Can you work these out from the model? Positions are in its coordinate system, mm. A direction names the side the tool comes from. Give positions to 0.01 mm unless a question says otherwise; leave off trailing zeros. Loops run counter-clockwise (first coordinate to the right, second up) from the corner with the lowest first, then second, coordinate; pieces in that order, holes last. Notation, with made-up numbers: (25, -3.75) - (79, -3.75) arc R27 cw to (79, 26.25) - close; hole circle Ø8 at (34.5, 0). An arc over 180 degrees is marked (long way). Answer as a JSON object with one key per item and string values.
```python
from build123d import *

# Parameters (mm, degrees)
EXTRUDE_1_DEPTH      = 8
SKETCH_2_R           = 2
CUT_EXTRUDE_1_DEPTH  = 8
SKETCH_3_W           = 235.5
SKETCH_3_H           = 139.5
CUT_EXTRUDE_2_DEPTH  = 6
SKETCH_4_R           = 2
CUT_EXTRUDE_3_DEPTH  = 6
SKETCH_6_W           = 6
SKETCH_6_H           = 6
SKETCH_6_R           = 2.1
EXTRUDE_2_DEPTH      = 4
SKETCH_7_R           = 24
SKETCH_7_R_2         = 21.5
EXTRUDE_3_DEPTH      = 3
SKETCH_8_R           = 2
CUT_EXTRUDE_4_DEPTH  = 3
SKETCH_9_W           = 11.5
SKETCH_9_H           = 15.5
CUT_EXTRUDE_5_DEPTH  = 7
CUT_EXTRUDE_6_DEPTH  = 6
SKETCH_11_W          = 20
SKETCH_11_H          = 26.5
CUT_EXTRUDE_8_DEPTH  = 1
SKETCH_13_W          = 26.5
SKETCH_13_H          = 5.5
CUT_EXTRUDE_9_DEPTH  = 5.25
SKETCH_14_W          = 9.2
SKETCH_14_H          = 3.5
SKETCH_14_W_2        = 7.8
SKETCH_14_H_2        = 1
CUT_EXTRUDE_10_DEPTH = 5.25
EXTRUDE_5_DEPTH      = 5.25
EXTRUDE_6_DEPTH      = 5.25
SKETCH_17_R          = 3
CUT_EXTRUDE_11_DEPTH = 2


with BuildPart() as part:
    # 草图1 → 凸台-拉伸1 (new body)
    with BuildSketch(Plane(origin=(0, 0, 0), x_dir=(1, 0, 0), z_dir=(0, 1, 0))):
        with BuildLine():
            Line((-106.707018927, 68.788249211), (123.292981073, 68.788249211))
            ThreePointArc((123.292981073, 68.788249211), (130.364048884, 65.859317023), (133.292981073, 58.788249211))
            Line((133.292981073, 58.788249211), (133.292981073, -80.961750789))
            ThreePointArc((133.292981073, -80.961750789), (130.364048884, -88.032818601), (123.292981073, -90.961750789))
            Line((123.292981073, -90.961750789), (-106.707018927, -90.961750789))
            ThreePointArc((-106.707018927, -90.961750789), (-113.778086739, -88.032818601), (-116.707018927, -80.961750789))
            Line((-116.707018927, -80.961750789), (-116.707018927, 58.788249211))
            ThreePointArc((-116.707018927, 58.788249211), (-113.778086739, 65.859317023), (-106.707018927, 68.788249211))
        make_face()
    extrude(amount=EXTRUDE_1_DEPTH)

    # 草图2 → 切除-拉伸1 (cut)
    with BuildSketch(Plane(origin=(0, 8, 0), x_dir=(1, 0, 0), z_dir=(0, 1, 0))):
        with Locations(Location((-103.707018927, 63.788249211, 0), (0, 0, 270))):
            Circle(SKETCH_2_R)
        with Locations(Location((-103.707018927, -85.961750789, 0), (0, 0, 270))):
            Circle(SKETCH_2_R)
        with Locations(Location((120.292981073, -85.961750789, 0), (0, 0, 270))):
            Circle(SKETCH_2_R)
        with Locations(Location((120.292981073, 63.788249211, 0), (0, 0, 270))):
            Circle(SKETCH_2_R)
    extrude(amount=-CUT_EXTRUDE_1_DEPTH, mode=Mode.SUBTRACT)

    # 草图3 → 切除-拉伸2 (cut)
    with BuildSketch(Plane(origin=(0, 8, 0), x_dir=(1, 0, 0), z_dir=(0, 1, 0))):
        with Locations((9.292981073, -11.211750789)):
            Rectangle(SKETCH_3_W, SKETCH_3_H)
    extrude(amount=-CUT_EXTRUDE_2_DEPTH, mode=Mode.SUBTRACT)

    # 草图4 → 切除-拉伸3 (cut)
    with BuildSketch(Plane(origin=(0, 2, 0), x_dir=(1, 0, 0), z_dir=(0, 1, 0))):
        with Locations(Location((-25.957018927, 40.538249211, 0), (0, 0, 270))):
            Circle(SKETCH_4_R)
        with Locations(Location((-7.957018927, 40.538249211, 0), (0, 0, 270))):
            Circle(SKETCH_4_R)
        with Locations(Location((10.042981073, 40.538249211, 0), (0, 0, 270))):
            Circle(SKETCH_4_R)
        with Locations(Location((28.042981073, 40.538249211, 0), (0, 0, 270))):
            Circle(SKETCH_4_R)
        with Locations(Location((50.042981073, 40.538249211, 0), (0, 0, 270))):
            Circle(SKETCH_4_R)
    extrude(amount=-CUT_EXTRUDE_3_DEPTH, mode=Mode.SUBTRACT)

    # 草图6 → 凸台-拉伸2 (add)
    # profile 1 of 3: a face of its own
    with BuildSketch(Plane(origin=(0, 2, 0), x_dir=(1, 0, 0), z_dir=(0, 1, 0))):
        with Locations((58.042981073, 40.538249211)):
            Rectangle(SKETCH_6_W, SKETCH_6_H)
        with Locations(Location((58.042981073, 40.538249211, 0), (0, 0, 270))):
            Circle(SKETCH_6_R, mode=Mode.SUBTRACT)
    # profile 2 of 3: a face of its own
    with BuildSketch(Plane(origin=(0, 2, 0), x_dir=(1, 0, 0), z_dir=(0, 1, 0))):
        with Locations((1.042981073, 40.538249211)):
            Rectangle(SKETCH_6_W, SKETCH_6_H)
        with Locations(Location((1.042981073, 40.538249211, 0), (0, 0, 270))):
            Circle(SKETCH_6_R, mode=Mode.SUBTRACT)
    # profile 3 of 3: a face of its own
    with BuildSketch(Plane(origin=(0, 2, 0), x_dir=(1, 0, 0), z_dir=(0, 1, 0))):
        with Locations((-34.957018927, 40.538249211)):
            Rectangle(SKETCH_6_W, SKETCH_6_H)
        with Locations(Location((-34.957018927, 40.538249211, 0), (0, 0, 270))):
            Circle(SKETCH_6_R, mode=Mode.SUBTRACT)
    extrude(amount=EXTRUDE_2_DEPTH)

    # 草图7 → 凸台-拉伸3 (add)
    # profile 1 of 2: a face of its own
    with BuildSketch(Plane(origin=(0, 2, 0), x_dir=(1, 0, 0), z_dir=(0, 1, 0))):
        with Locations(Location((-76.707018927, 28.788249211, 0), (0, 0, 270))):
            Circle(SKETCH_7_R)
        with Locations(Location((-76.707018927, 28.788249211, 0), (0, 0, 270))):
            Circle(SKETCH_7_R_2, mode=Mode.SUBTRACT)
    # profile 2 of 2: a face of its own
    with BuildSketch(Plane(origin=(0, 2, 0), x_dir=(1, 0, 0), z_dir=(0, 1, 0))):
        with Locations(Location((93.292981073, 28.788249211, 0), (0, 0, 270))):
            Circle(SKETCH_7_R)
        with Locations(Location((93.292981073, 28.788249211, 0), (0, 0, 270))):
            Circle(SKETCH_7_R_2, mode=Mode.SUBTRACT)
    extrude(amount=EXTRUDE_3_DEPTH)

    # 草图8 → 切除-拉伸4 (cut)
    with BuildSketch(Plane(origin=(0, 2, 0), x_dir=(1, 0, 0), z_dir=(0, 1, 0))):
        with Locations(Location((-82.480521619, 38.788249211, 0), (0, 0, 270))):
            Circle(SKETCH_8_R)
        with Locations(Location((-70.933516236, 38.788249211, 0), (0, 0, 270))):
            Circle(SKETCH_8_R)
        with Locations(Location((-65.160013544, 28.788249211, 0), (0, 0, 270))):
            Circle(SKETCH_8_R)
        with Locations(Location((-70.933516236, 18.788249211, 0), (0, 0, 270))):
            Circle(SKETCH_8_R)
        with Locations(Location((-82.480521619, 18.788249211, 0), (0, 0, 270))):
            Circle(SKETCH_8_R)
        with Locations(Location((-88.254024311, 28.788249211, 0), (0, 0, 270))):
            Circle(SKETCH_8_R)
        with Locations(Location((87.519478381, 38.788249211, 0), (0, 0, 270))):
            Circle(SKETCH_8_R)
        with Locations(Location((99.066483764, 38.788249211, 0), (0, 0, 270))):
            Circle(SKETCH_8_R)
        with Locations(Location((104.839986456, 28.788249211, 0), (0, 0, 270))):
            Circle(SKETCH_8_R)
        with Locations(Location((99.066483764, 18.788249211, 0), (0, 0, 270))):
            Circle(SKETCH_8_R)
        with Locations(Location((87.519478381, 18.788249211, 0), (0, 0, 270))):
            Circle(SKETCH_8_R)
        with Locations(Location((81.745975689, 28.788249211, 0), (0, 0, 270))):
            Circle(SKETCH_8_R)
    extrude(amount=-CUT_EXTRUDE_4_DEPTH, mode=Mode.SUBTRACT)

    # 草图9 → 切除-拉伸5 (cut)
    with BuildSketch(Plane(origin=(0, 8, 0), x_dir=(1, 0, 0), z_dir=(0, 1, 0))):
        with Locations((127.542981073, -43.211750789)):
            Rectangle(SKETCH_9_W, SKETCH_9_H)
    extrude(amount=-CUT_EXTRUDE_5_DEPTH, mode=Mode.SUBTRACT)

    # 草图10 → 切除-拉伸6 (cut)
    with BuildSketch(Plane(origin=(0, 8, 0), x_dir=(1, 0, 0), z_dir=(0, 1, 0))):
        Polygon((127.042981073, 33.788249211), (127.042981073, 22.788249211), (129.792981073, 22.788249211), (129.792981073, 17.788249211), (130.792981073, 17.788249211), (130.792981073, 24.788249211), (133.292981073, 24.788249211), (133.292981073, 31.788249211), (130.792981073, 31.788249211), (130.792981073, 38.788249211), (129.792981073, 38.788249211), (129.792981073, 33.788249211), align=None)
    extrude(amount=-CUT_EXTRUDE_6_DEPTH, mode=Mode.SUBTRACT)

    # 草图11 → 切除-拉伸8 (cut)
    with BuildSketch(Plane(origin=(0, 2, 0), x_dir=(1, 0, 0), z_dir=(0, 1, 0))):
        with Locations((122.292981073, -10.461750789)):
            Rectangle(SKETCH_11_W, SKETCH_11_H)
    extrude(amount=-CUT_EXTRUDE_8_DEPTH, mode=Mode.SUBTRACT)

    # 草图13 → 切除-拉伸9 (cut)
    with BuildSketch(Plane.ZY.offset(-127.042981073)):
        with Locations((10.461750789, 4.75)):
            Rectangle(SKETCH_13_W, SKETCH_13_H)
    extrude(amount=-CUT_EXTRUDE_9_DEPTH, mode=Mode.SUBTRACT)

    # 草图14 → 切除-拉伸10 (cut)
    with BuildSketch(Plane.ZY.offset(-132.292981073)):
        with Locations((15.611750789, 4.25)):
            Rectangle(SKETCH_14_W, SKETCH_14_H)
        with Locations((4.111750789, 3)):
            Rectangle(SKETCH_14_W_2, SKETCH_14_H_2)
    extrude(amount=-CUT_EXTRUDE_10_DEPTH, mode=Mode.SUBTRACT)

    # 草图15 → 凸台-拉伸5 (add)
    with BuildSketch(Plane.ZY.offset(-127.042981073)):
        Polygon((-2.788249211, 7.5), (-0.288249211, 7.5), (-2.788249211, 5), align=None)
    extrude(amount=-EXTRUDE_5_DEPTH)

    # 草图16 → 凸台-拉伸6 (add)
    with BuildSketch(Plane.ZY.offset(-127.042981073)):
        Polygon((23.711750789, 7.5), (23.711750789, 5.5), (21.711750789, 7.5), align=None)
    extrude(amount=-EXTRUDE_6_DEPTH)

    # 草图17 → 切除-拉伸11 (cut)
    with BuildSketch(Plane.XZ):
        with Locations(Location((-103.707018927, 85.961750789, 0), (0, 0, 270))):
            Circle(SKETCH_17_R)
        with Locations(Location((120.292981073, 85.961750789, 0), (0, 0, 270))):
            Circle(SKETCH_17_R)
        with Locations(Location((120.292981073, -63.788249211, 0), (0, 0, 270))):
            Circle(SKETCH_17_R)
        with Locations(Location((-103.707018927, -63.788249211, 0), (0, 0, 270))):
            Circle(SKETCH_17_R)
    extrude(amount=-CUT_EXTRUDE_11_DEPTH, mode=Mode.SUBTRACT)


solid = part.part
```
1) Imagine slicing it at B-B on x = -14.5. Write out the boundary of the cut face in (y, z), and give its area (3 significant figures).
Check sheet entries:
{"outline": "(0, -68.79) - (8, -68.79) - (8, -58.54) - (2, -58.54) - (2, 80.96) - (8, 80.96) - (8, 90.96) - (0, 90.96) - close", "area": "441 mm2"}
2) Imagine slicing it at C-C on x = -93. Write out the boundary of the cut face in (y, z), and give its area (3 significant figures).
Check sheet entries:
{"outline": "(0, -68.79) - (8, -68.79) - (8, -58.54) - (2, -58.54) - (2, -46.41) - (5, -46.41) - (5, -42.82) - (2, -42.82) - (2, -14.76) - (5, -14.76) - (5, -11.17) - (2, -11.17) - (2, 80.96) - (8, 80.96) - (8, 90.96) - (0, 90.96) - close", "area": "463 mm2"}
3) If we mould it in two halves opening along Z, with no side actions, what happens to faces 4 (the flat face through (57, 6, -43)), 5 (the flat face through (-116.707, 4, 12)), 6 (the cylindrical face through (-113.855, 3.944, -65.781))? For each: released by +Z, released by -Z, zero draft, split by the parting line, or undercut.
Check sheet entries:
{"face 4": "undercut", "face 5": "zero draft", "face 6": "released by -Z"}
4) I'm going to push flat-ended pins straight in: P1, Ø4.5, axis at x = -65.16, z = -28.79, coming from the +Y side; P2, Ø3, axis at x = -103.5, z = -63.5, coming from the -Y side; P3, Ø3.5, axis at x = 130, z = 42.5, coming from the +Y side. Where does each tip first touch, or does it pass through?
Check sheet entries:
{"P1": "y = 2", "P2": "through", "P3": "y = 1"}
5) I need wall thicknesses on L1, parallel to Z at x = -35, y = 2.5; L2, parallel to Z at x = -84, y = 7; L3, parallel to X at y = 7.75, z = 30.5. Which ranges of each line are inside material? Lowest first, please.
Check sheet entries:
{"L1": "-68.79 to -58.54, -43.54 to -42.64, -38.44 to -37.54, 80.96 to 90.96", "L2": "-68.79 to -58.54, 80.96 to 90.96", "L3": "-116.71 to -108.46, 127.04 to 133.29"}
6) Imagine slicing it at A-A on z = 68. Write out the boundary of the cut face in (x, y).
Check sheet entries:
{"outline": "(-116.71, 0) - (133.29, 0) - (133.29, 8) - (127.04, 8) - (127.04, 2) - (-108.46, 2) - (-108.46, 8) - (-116.71, 8) - close"}
7) Which directions (+Z, -Z, +X, -X, +Y, -Y) give clear straight access to the entire face, cutting with the end or side of a thin tool? Please do faces 1 (the flat face through (130, 5, 50.962)), 2 (the flat face through (130.793, 5, -21)), 3 (the flat face through (132.293, 4.3, 10.6)).
Check sheet entries:
{"face 1": "+X, +Y", "face 2": "+Y", "face 3": "none"}
